from build123d import *

# Parameters (mm, degrees)
SKETCH1_R           = 9
BOSS_EXTRUDE1_DEPTH = 3.175
BOSS_EXTRUDE2_DEPTH = 11
SKETCH3_R           = 6.5
BOSS_EXTRUDE3_DEPTH = 2
SKETCH4_R           = 4.5
BOSS_EXTRUDE4_DEPTH = 5
BOSS_EXTRUDE5_DEPTH = 3.175
BOSS_EXTRUDE7_DEPTH = 3.175
SKETCH8_R           = 2
CUT_EXTRUDE1_DEPTH  = 11.35


with BuildPart() as part:
    # Sketch1 → Boss-Extrude1 (new body)
    with BuildSketch(Plane(origin=(0, 0, 0), x_dir=(1, 0, 0), z_dir=(0, 1, 0))):
        Circle(SKETCH1_R)
    extrude(amount=BOSS_EXTRUDE1_DEPTH)

    # Sketch2 → Boss-Extrude2 (add)
    with BuildSketch(Plane(origin=(0, 3.175, 0), x_dir=(1, 0, 0), z_dir=(0, 1, 0))):
        with BuildLine():
            Line((-7.707704384, -4.646643211), (-5.138469589, -3.097762141))
            ThreePointArc((-5.138469589, -3.097762141), (0, 6), (5.138469589, -3.097762141))
            Line((5.138469589, -3.097762141), (7.707704384, -4.646643211))
            ThreePointArc((7.707704384, -4.646643211), (0, 9), (-7.707704384, -4.646643211))
        make_face()
    extrude(amount=BOSS_EXTRUDE2_DEPTH)

    # Sketch3 → Boss-Extrude3 (add)
    with BuildSketch(Plane.XZ):
        Circle(SKETCH3_R)
    extrude(amount=BOSS_EXTRUDE3_DEPTH)

    # Sketch4 → Boss-Extrude4 (add)
    with BuildSketch(Plane.XZ.offset(2)):
        Circle(SKETCH4_R)
    extrude(amount=BOSS_EXTRUDE4_DEPTH)

    # Sketch6 → Boss-Extrude5 (add)
    with BuildSketch(Plane(origin=(0, 0, 0), x_dir=(1, 0, 0), z_dir=(0, 1, 0))):
        with BuildLine():
            Line((-9, 0), (-9, 13.194197425))
            ThreePointArc((-9, 13.194197425), (-4.5, 17.694197425), (0, 13.194197425))
            Line((0, 13.194197425), (0, 9))
            ThreePointArc((0, 9), (-6.363961031, 6.363961031), (-9, 0))
        make_face()
    extrude(amount=BOSS_EXTRUDE5_DEPTH)

    # Sketch7 → Boss-Extrude7 (add)
    with BuildSketch(Plane(origin=(0, 8.174999906, 0), x_dir=(1, 0, 0), z_dir=(0, 1, 0))):
        with BuildLine():
            Line((0, 9), (0, 13.194197425))
            ThreePointArc((0, 13.194197425), (-4.5, 17.694197425), (-9, 13.194197425))
            Line((-9, 13.194197425), (-9, 0))
            ThreePointArc((-9, 0), (-6.363961031, 6.363961031), (0, 9))
        make_face()
    extrude(amount=BOSS_EXTRUDE7_DEPTH)

    # Sketch8 → Cut-Extrude1 (cut)
    with BuildSketch(Plane(origin=(0, 11.349999906, 0), x_dir=(1, 0, 0), z_dir=(0, 1, 0))):
        with Locations((-4.5, 13.194197425)):
            Circle(SKETCH8_R)
    extrude(amount=-CUT_EXTRUDE1_DEPTH, mode=Mode.SUBTRACT)


solid = part.part
Could you check a few things on this model? Use its own coordinates, in mm. A direction names the side the tool comes from. Coordinates: 2 decimals unless noted, no trailing zeros. Loops run counter-clockwise (first coordinate to the right, second up) from the corner with the lowest first, then second, coordinate; pieces in that order, holes last. Notation, with made-up numbers: (-36, 32) -> (15, 32) arc R10 cw to (15, 47) -> close; hole circle Ø2 at (27, -34.75). An arc over 180 degrees is marked (long way). Answer in a Markdown table with one row per item.
(1) Imagine slicing it at B-B (z = -7). List the corners of the cut face in (x, y) for me (3 decimals).
Results found:
| item | result |
|---|---|
| outline | (-9, 0) -> (5.657, 0) -> (5.657, 14.175) -> (-5.657, 14.175) -> (-5.657, 11.35) -> (-9, 11.35) -> (-9, 8.175) -> (-5.657, 8.175) -> (-5.657, 3.175) -> (-9, 3.175) -> close |
(2) Thinking about a two-plate mould opening in X: for faces 4 (the face through (6.405, 8.598, 3.861)), 5 (the face through (0, 2, -11)), 6 (the face through (-4.599, 1.565, -17.693)), 7 (the face through (-2, 0, -7)), which applies, released by +X, released by -X, zero draft, split by the parting line, or undercut?
Results found:
| item | result |
|---|---|
| face 4 | undercut |
| face 5 | released by +X |
| face 6 | split by the parting line |
| face 7 | zero draft |
(3) Will these pins go through, and if not, where does the flat tip stop? pin 1 Ø1.6 at (y, z) = (2, -10.5) entering from +X; pin 2 Ø4 at (x, y) = (3, 0.5) entering from -Z; pin 3 Ø9.5 at (x, z) = (0, 0) entering from +Y (3 decimals); pin 4 Ø2.5 at (x, z) = (-4.5, -13.19) entering from -Y.
Results found:
| item | result |
|---|---|
| pin 1 | stops at x = 0 |
| pin 2 | stops at z = -8.94 |
| pin 3 | stops at y = 3.175 |
| pin 4 | passes through |
(4) Imagine slicing it at C-C (x = 1). List the corners of the cut face in (y, z) for me (3 decimals).
Results found:
| item | result |
|---|---|
| outline | (-7, -4.387) -> (-2, -4.387) -> (-2, -6.423) -> (0, -6.423) -> (0, -8.944) -> (14.175, -8.944) -> (14.175, -5.916) -> (3.175, -5.916) -> (3.175, 8.944) -> (0, 8.944) -> (0, 6.423) -> (-2, 6.423) -> (-2, 4.387) -> (-7, 4.387) -> close |
(5) For faces 1 (the face through (0, 9, -6)), 2 (the face through (-4.42, -2, 1.54)), 3 (the face through (0, 10, -11)), which set-ups out of +Z, -Z, +X, -X, +Y, -Y let a thin tool reach every point of the face, with its end or its side?
Results found:
| item | result |
|---|---|
| face 1 | +Y |
| face 2 | -Y |
| face 3 | -Z, +X, +Y, -Y |
(6) Imagine slicing it at A-A (x = -4). List the corners of the cut face in (y, z) for me (3 decimals).
Results found:
| item | result |
|---|---|
| outline | (-7, -2.062) -> (-2, -2.062) -> (-2, -5.123) -> (0, -5.123) -> (0, -11.258) -> (3.175, -11.258) -> (3.175, -8.062) -> (8.175, -8.062) -> (8.175, -11.258) -> (11.35, -11.258) -> (11.35, -8.062) -> (14.175, -8.062) -> (14.175, -4.472) -> (3.175, -4.472) -> (3.175, 8.062) -> (0, 8.062) -> (0, 5.123) -> (-2, 5.123) -> (-2, 2.062) -> (-7, 2.062) -> close; (0, -17.666) -> (3.175, -17.666) -> (3.175, -15.131) -> (0, -15.131) -> close; (8.175, -17.666) -> (11.35, -17.666) -> (11.35, -15.131) -> (8.175, -15.131) -> close |
(7) If I drill on probe 1 along Y at (x, z) = (-4.25, -10.5) (3 decimals); probe 2 along X at (y, z) = (9.5, 0); probe 3 along Y at (x, z) = (6, -6) (3 decimals), over which ranges is the centre line in solid material (lowest first)?
Results found:
| item | result |
|---|---|
| probe 1 | y = 0 to 3.175, 8.175 to 11.35 |
| probe 2 | x = -9 to -6, 6 to 9 |
| probe 3 | y = 0 to 14.175 |
